For this review, take the finished solid that the model builds, in its own axes (mm). A direction names the side the tool comes from. Give positions to 0.01 mm unless a question says otherwise; leave off trailing zeros. Loops run counter-clockwise (first coordinate to the right, second up) from the corner with the lowest first, then second, coordinate; pieces in that order, holes last.
Autodesk Inventor part; units mm, degrees
ref_plane "YZ Plane" through (0, 0, 0) normal (1, 0, 0) x (0, 1, 0)
ref_plane "XZ Plane" through (0, 0, 0) normal (0, 1, 0) x (-1, 0, 0)
ref_plane "XY Plane" through (0, 0, 0) normal (0, 0, 1) x (1, 0, 0)
sketch "Sketch1" plane through (0, 0, 0) normal (0, 0, 1) x (1, 0, 0)
  line L0 (-131.0833, 65.4113) -> (124.5042, 65.4113)
  line L1 (124.5042, 65.4113) -> (124.5042, -0.7128)
  line L2 (124.5042, -0.7128) -> (-131.0833, -0.7128)
  line L3 (-131.0833, -0.7128) -> (-131.0833, 65.4113)
  point P0 (0, 0)
extrude "Extrusion1" add sketch "Sketch1" along normal blind 6.35
ref_plane "Work Plane2" through (124.5042, 65.4113, 3.175) normal (1, 0, 0) x (0, 0, -1)
sketch "Sketch4" plane through (124.5042, 65.4113, 3.175) normal (1, 0, 0) x (0, 0, -1)
  line L0 (3.175, -66.1241) -> (3.175, 0)
  line L1 (3.175, -66.1241) -> (69.85, -66.1241)
  line L2 (69.85, -66.1241) -> (69.85, 0)
  line L3 (69.85, 0) -> (3.175, 0)
  line L4 (3.175, 0) -> (3.175, -66.1241)
  point P0 (3.175, -65.4113)
  dimension "d2" = 66.1241
  dimension "d3" = 66.675
extrude "Extrusion2" add sketch "Sketch4" against normal blind 6.35
fillet "Fillet1" radius 44.45 1 edges at (121.3292, -0.7128, -66.675)
ref_plane "Work Plane3" through (-131.0833, -0.7128, 0) normal (-1, 0, 0) x (0, 0, 1)
sketch "Sketch5" plane through (-131.0833, -0.7128, 0) normal (-1, 0, 0) x (0, 0, 1)
  line L0 (0, 66.1241) -> (-66.675, 66.1241)
  line L1 (0, 66.1241) -> (-66.675, 66.1241)
  line L2 (-66.675, 66.1241) -> (-66.675, 0)
  line L3 (-66.675, 0) -> (0, 0)
  line L4 (0, 0) -> (0, 66.1241)
  point P0 (0, 0.7128)
extrude "Extrusion3" add sketch "Sketch5" against normal blind 6.35
fillet "Fillet2" radius 44.45 1 edges at (-127.9083, -0.7128, -66.675)
ref_plane "Work Plane4" through (118.1542, 65.4113, -66.675) normal (-1, 0, 0) x (0, 0, 1)
sketch "Sketch6" plane through (118.1542, 65.4113, -66.675) normal (-1, 0, 0) x (0, 0, 1)
  circle A0 centre (60.325, -12.7) radius 1.5875
  point P0 (66.675, -65.4113)
  dimension "d11" = 3.175
extrude "Extrusion4" add sketch "Sketch6" along normal blind 5.08
properties part number "Top Basic layout"
Item 1: For L1, parallel to X at y = 61, z = -14; L2, parallel to Z at x = -106.5, y = 48, list the stretches that pass through material, from the lowest coordinate up.
Answer:
L1: x = -131.08 to -124.73, 118.15 to 124.5
L2: z = 0 to 6.35
Item 2: Take a section at C-C on x = 66.5. Give the boundary of the cut face in (y, z), and give its area (3 significant figures).
Answer:
outline: (-0.71, 0) - (65.41, 0) - (65.41, 6.35) - (-0.71, 6.35) - close
area: 420 mm2
Item 3: Tool access review of faces 1 (the flat face through (-128, 55, -66.675)), 2 (the flat face through (-124.733, 33, -34)): name each direction out of +Z, -Z, +X, -X, +Y, -Y from which nothing blocks a thin tool from reaching the whole face with its end or side.
Answer:
face 1: -Z, +X, -X, +Y, -Y
face 2: -Z, +Y, -Y
Item 4: Clearance check with a flat-ended pin moving along its axis: pin 1 Ø1.5 at (x, y) = (89, 25) entering from -Z. State where the tip first meets the part, or that it passes through.
Answer:
pin 1: stops at z = 0
Item 5: Take a section at A-A on z = -57. Give the boundary of the cut face in (x, y).
Answer:
outline: (-131.08, 16.05) - (-124.73, 16.05) - (-124.73, 65.41) - (-131.08, 65.41) - close; (118.15, 16.05) - (124.5, 16.05) - (124.5, 65.41) - (118.15, 65.41) - close
Item 6: The part is to be moulded in two halves that separate along X. For faces 3 (the flat face through (118.154, 33, -33)), 4 (the flat face through (-5, 33, 6.35)), 5 (the flat face through (124.504, 33, -31)), say which applies: released by +X, released by -X, zero draft, split by the parting line, or undercut.
Answer:
face 3: undercut
face 4: zero draft
face 5: released by +X
Item 7: Take a section at B-B on y = 29. Give the boundary of the cut face in (x, z), and give its area (3 significant figures).
Answer:
outline: (-131.08, -64.16) - (-124.73, -64.16) - (-124.73, 0) - (118.15, 0) - (118.15, -64.16) - (124.5, -64.16) - (124.5, 6.35) - (-131.08, 6.35) - close
area: 2,440 mm2
